Build history of the part. All positions in model axes, mm. Face numbers are marked on the shaded views. Give positions to 0.01 mm unless a question says otherwise; leave off trailing zeros. Loops run counter-clockwise (first coordinate to the right, second up) from the corner with the lowest first, then second, coordinate; pieces in that order, holes last. Notation, with made-up numbers: M 82.5,-8.75 L 88.5,-8.75 A27 ccw 88.5,14.25 Z; hole C -30.5,22 d2. An arc over 180 degrees is marked long. Put each result on its own line as item: value.
```python
from build123d import *

# Parameters (mm, degrees)
F1_W     = 55
F1_H     = 45
F2_DEPTH = 3
F0_W     = 60
F0_H     = 50
F3_DEPTH = 1


with BuildPart() as f2:
    # F1 (on face) → F2 (new body)
    with BuildSketch(Plane.XZ):
        Rectangle(F1_W, F1_H)
    extrude(amount=F2_DEPTH)

    # F0 (on Front) → F3 (join)
    with BuildSketch(Plane.XZ):
        Rectangle(F0_W, F0_H)
    extrude(amount=F3_DEPTH)


solid = f2.part
```
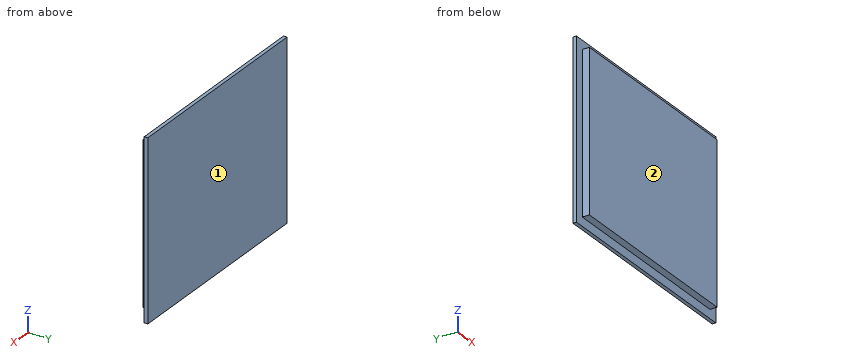
Q1. Probe line 1 (X direction, y = -1.8, z = 15); line 2 (Z direction, x = -18, y = -2.45); line 3 (Y direction, x = 28, z = -13.5). List the from-to ranges inside material, lowest first. Write a range as from..to.
Here are the results:
line 1: -27.5..27.5
line 2: -22.5..22.5
line 3: -1..0
Q2. Slice it at B-B (x = 11). List the corners of the cut face in (y, z), and give its area (3 significant figures).
Here are the results:
outline: M -3,-22.5 L -1,-22.5 L -1,-25 L 0,-25 L 0,25 L -1,25 L -1,22.5 L -3,22.5 Z
area: 140 mm²
Q3. Slice it at C-C (y = -2). List the corners of the cut face in (x, z), and give its area (4 significant figures).
Here are the results:
outline: M -27.5,-22.5 L 27.5,-22.5 L 27.5,22.5 L -27.5,22.5 Z
area: 2,475 mm²
Q4. Drop a flat-ended pin along its axis: pin 1 Ø1 at (y, z) = (-2, -16.5) entering from -X. Give the stop position or say it passes through.
Here are the results:
pin 1: x = -27.5
Q5. Slice it at A-A (z = 5). List the corners of the cut face in (x, y), and give its area (3 significant figures).
Here are the results:
outline: M -30,-1 L -27.5,-1 L -27.5,-3 L 27.5,-3 L 27.5,-1 L 30,-1 L 30,0 L -30,0 Z
area: 170 mm²
Q6. Mould opens along Y. For the marked faces 1 and 2 say: pulls with the +Y half, pulls with the -Y half, needs draft (parallel to the pull), parting line crosses it, or undercut.
Here are the results:
face 1: pulls with the +Y half
face 2: pulls with the -Y half
